Geometry: see drawing. Coordinates: mm, zero at the bounding-box minimum. A direction names the side the tool comes from. Give positions to 0.01 mm unless a question says otherwise; leave off trailing zeros. Loops run counter-clockwise (first coordinate to the right, second up) from the corner with the lowest first, then second, coordinate; pieces in that order, holes last. Notation, with made-up numbers: (49, 15) -> (86, 15) arc R12 cw to (86, 21) -> close; hole circle Ø8 at (78.25, 82.25). An arc over 180 degrees is marked (long way). Return JSON: item names as keys, results as strings. Group by question number.
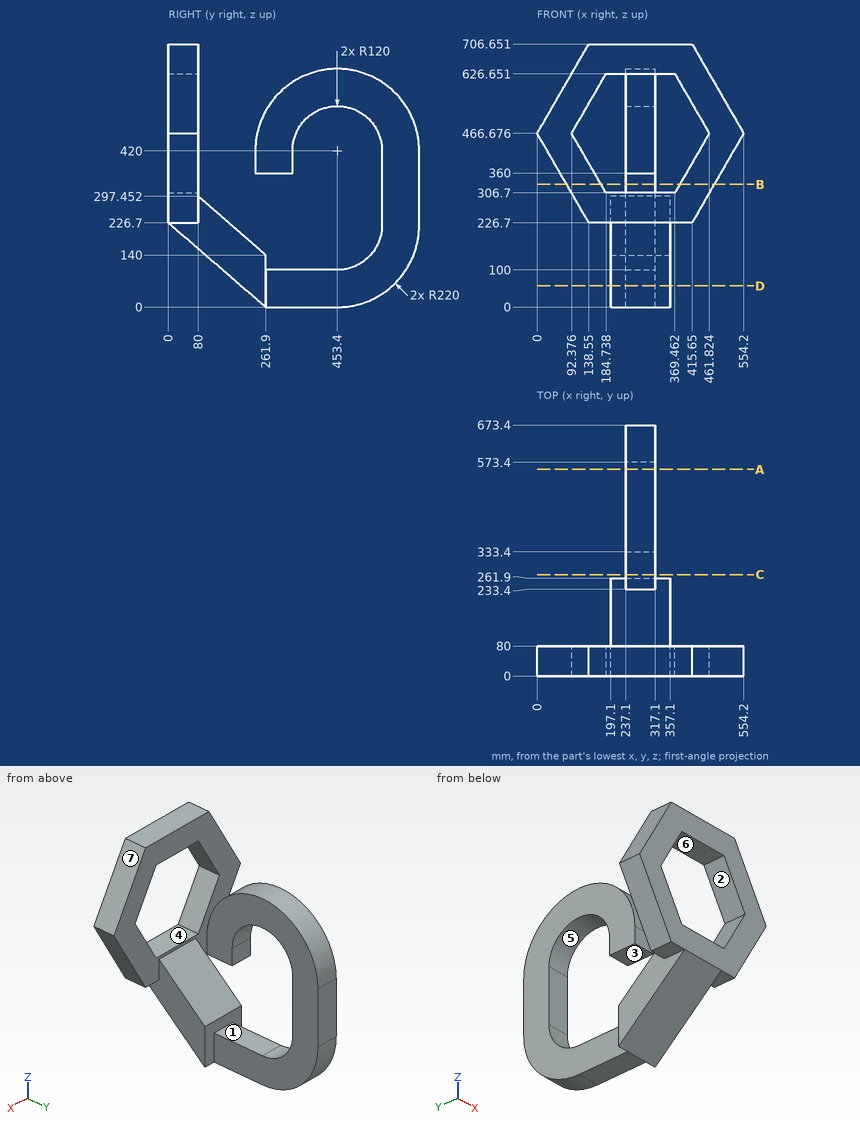
1) Cut plane C-C on y = 272. Return loops of the section in (x, z) (1 decimal).
2) Reachability of the marked faces 1, 2, 3 and 4 from +Z, -Z, +X, -X, +Y, -Y: full face, straight path, thin tool, end or side. Return the list, or none.
3) Mould query, pull axis X, two halves, no side actions, for the marked faces 5, 6 and 7. Classes: released by +X, released by -X, zero draft, split by the parting line, or undercut.
4) Material intervals for line 1 (Y direction, x = 402, z = 312); line 2 (X direction, y = 485, z = 60.5); line 3 (Y direction, x = 302, z = 364.5), sorted ascending.
5) Cut plane B-B on z = 330. Return loops of the section in (x, y).
6) Contact query for flat-ended pins moving along their axis: P1, Ø1, axis at x = 253.5, z = 182.5, coming from the +Y side; P2, Ø24, axis at x = 282, y = 285, coming from the -Z side; P3, Ø1.5, axis at x = 211, z = 110, coming from the -Y side (1 decimal). Output: stop coordinate, or through.
7) Cut plane A-A on y = 555. Return loops of the section in (x, z) (1 decimal), then the cut area to 3 significant figures.
8) Cut plane D-D on z = 57. Return loops of the section in (x, y), then the cut area to 3 significant figures.
Calculated:
{
 "1": {"outline": "(237.1, 0) -> (317.1, 0) -> (317.1, 100) -> (237.1, 100) -> close; (237.1, 360) -> (317.1, 360) -> (317.1, 544.5) -> (237.1, 544.5) -> close"},
 "2": {"face 1": "+X, -X", "face 2": "+Y, -Y", "face 3": "+X, -X, -Y", "face 4": "-Y"},
 "3": {"face 5": "zero draft", "face 6": "undercut", "face 7": "released by +X"},
 "4": {"line 1": "0 to 80", "line 2": "237.1 to 317.1", "line 3": "233.4 to 333.4, 573.4 to 673.4"},
 "5": {"outline": "(78.91, 0) -> (171.29, 0) -> (171.29, 80) -> (78.91, 80) -> close; (237.1, 573.4) -> (317.1, 573.4) -> (317.1, 673.4) -> (237.1, 673.4) -> close; (382.91, 0) -> (475.29, 0) -> (475.29, 80) -> (382.91, 80) -> close"},
 "6": {"P1": "y = 670.27", "P2": "z = 0", "P3": "y = 134"},
 "7": {"outline": "(237.1, 24.9) -> (317.1, 24.9) -> (317.1, 156.1) -> (237.1, 156.1) -> close; (237.1, 483.9) -> (317.1, 483.9) -> (317.1, 615.1) -> (237.1, 615.1) -> close", "area": "21,000 mm2"},
 "8": {"outline": "(197.1, 196.05) -> (357.1, 196.05) -> (357.1, 261.9) -> (317.1, 261.9) -> (317.1, 601.15) -> (237.1, 601.15) -> (237.1, 261.9) -> (197.1, 261.9) -> close", "area": "37,700 mm2"}
}
